Work out the finished part from the listing and answer in its coordinate system (mm). A direction names the side the tool comes from. Round coordinates to 2 decimals unless told otherwise and drop trailing zeros. Loops run counter-clockwise (first coordinate to the right, second up) from the corner with the lowest first, then second, coordinate; pieces in that order, holes last.
from build123d import *

# Parameters (mm, degrees)
BOSS_EXTRUDE1_DEPTH = 20
BOSS_EXTRUDE2_DEPTH = 20


with BuildPart() as part:
    # Sketch1 → Boss-Extrude1 (new body)
    with BuildSketch(Plane.XY):
        Polygon((-15.2, -15.2), (-15.2, -3.885), (-13.2, -1.885), (-17.2, -1.885), (-17.2, -17.2), (17.2, -17.2), (17.2, -1.885), (13.2, -1.885), (13.2, -3.885), (15.2, -3.885), (15.2, -15.2), align=None)
    extrude(amount=BOSS_EXTRUDE1_DEPTH)

    # Sketch2 → Boss-Extrude2 (add)
    with BuildSketch(Plane(origin=(0, 0, 0), x_dir=(-1, 0, 0), z_dir=(0, 0, -1))):
        Polygon((-45, 50), (-17.2, -1.885), (-17.2, -6.119772924), (-31.226415692, 20.058665139), (-34.89374, 18.093711573), (-17.2, -13.142164629), (-17.2, -17.2), (-53, 46), (-53, 50), (-51.2, 50), (-51.2, 45.8), (-48.8, 45.8), (-48.8, 50), align=None)
        Polygon((-46.197392065, 48), (-32.170976373, 21.821561937), (-35.879759796, 19.834394564), (-47, 39.4656566), (-47, 48), align=None, mode=Mode.SUBTRACT)
    extrude(amount=-BOSS_EXTRUDE2_DEPTH)


solid = part.part
Item 1: For faces 1 (the face through (52, 50, 10)), 2 (the face through (47, 44, 10)), 3 (the face through (13.2, -3, 10)), determine the directions among +Z, -Z, +X, -X, +Y, -Y from which every point of the face is accessible in a straight line to the end or side of a thin tool.
Item 2: Determine the mould class of faces 4 (the face through (51.2, 48, 10)), 5 (the face through (-17.2, -9, 10)), 6 (the face through (26, 12, 0)) for opening direction X: pulls with the +X half, pulls with the -X half, needs draft (parallel to the pull), parting line crosses it, or undercut.
Item 3: Section C-C, the plane y = 26 is taken. Give the vertices of the cut face in (x, z), plus the area to 3 significant figures.
Item 4: Each of these flat-tipped pins is pushed along its axis until it touches: P1, Ø6, axis at y = 9.5, z = 7.5, coming from the +X side; P2, Ø2, axis at x = -9, z = 6.5, coming from the +Y side; P3, Ø2, axis at y = 48, z = 11, coming from the -X side. Where does it stop, or does it pass through?
Item 5: Straight lines are drawn through the part: line 1 (X direction, y = -10, z = 10.5); line 2 (X direction, y = -6, z = 5.25); line 3 (Y direction, x = 32.5, z = 17). For each, find the intervals that lie inside material, in ascending order.
Item 6: Section B-B, the plane y = -7 is taken. Give the vertices of the cut face in (x, z).
Item 7: Section A-A, the plane z = 11.25 is taken. Give the vertices of the cut face in (x, y) (3 decimals).
Item 8: Section D-D, the plane x = 24 is taken. Give the vertices of the cut face in (y, z).
Answer below:
1. face 1: +Z, -Z, +X, -X, +Y
1. face 2: +Z, -Z
1. face 3: +Z, -Z, +Y
2. face 4: undercut
2. face 5: pulls with the -X half
2. face 6: needs draft
3. outline: (32.14, 0) - (34.41, 0) - (34.41, 20) - (32.14, 20) - close; (39.37, 0) - (41.67, 0) - (41.67, 20) - (39.37, 20) - close
3. area: 91.4 mm2
4. P1: stops at x = 34.02
4. P2: stops at y = -15.2
4. P3: stops at x = 43.39
5. line 1: x = -17.2 to -15.2, 15.2 to 17.2, 18.98 to 21.28
5. line 2: x = -17.2 to -15.2, 15.2 to 17.26, 21.25 to 23.54
5. line 3: y = 9.81 to 13.87, 19.38 to 21.65, 22.44 to 26.67
6. outline: (-17.2, 0) - (-15.2, 0) - (-15.2, 20) - (-17.2, 20) - close; (15.2, 0) - (17.2, 0) - (17.2, 20) - (15.2, 20) - close; (20.68, 0) - (22.98, 0) - (22.98, 20) - (20.68, 20) - close
7. outline: (-17.2, -17.2) - (17.2, -17.2) - (53, 46) - (53, 50) - (51.2, 50) - (51.2, 45.8) - (48.8, 45.8) - (48.8, 50) - (45, 50) - (17.2, -1.885) - (13.2, -1.885) - (13.2, -3.885) - (15.2, -3.885) - (15.2, -15.2) - (-15.2, -15.2) - (-15.2, -3.885) - (-13.2, -1.885) - (-17.2, -1.885) - close; hole (17.2, -13.142) - (34.894, 18.094) - (31.226, 20.059) - (17.2, -6.12) - close; hole (32.171, 21.822) - (35.88, 19.834) - (47, 39.466) - (47, 48) - (46.197, 48) - close
8. outline: (-5.2, 0) - (-1.14, 0) - (-1.14, 20) - (-5.2, 20) - close; (6.57, 0) - (10.81, 0) - (10.81, 20) - (6.57, 20) - close
